from build123d import *

# Parameters (mm, degrees)
BASE_FLANGE1_DEPTH              = 0.254
EDGE_FLANGE1_STRIP_W            = 1.0668
EDGE_FLANGE1_STRIP_H            = 0.254
EDGE_FLANGE1_STRIP_CUT_DEPTH    = 6.985
EDGE_FLANGE1_RELIEF_W           = 1.1938
EDGE_FLANGE1_RELIEF_H           = 0.127
EDGE_FLANGE1_RELIEF_CUT_DEPTH   = 0.254
EDGE_FLANGE1_DEPTH              = 6.985
EDGE_FLANGE2_STRIP_W            = 1.0668
EDGE_FLANGE2_STRIP_H            = 0.254
EDGE_FLANGE2_STRIP_CUT_DEPTH    = 8.244248495
EDGE_FLANGE2_RELIEF_W           = 1.1938
EDGE_FLANGE2_RELIEF_H           = 0.127
EDGE_FLANGE2_RELIEF_CUT_DEPTH   = 0.254
EDGE_FLANGE2_STRIP_2_W          = 1.0668
EDGE_FLANGE2_STRIP_2_H          = 0.254
EDGE_FLANGE2_STRIP_CUT_2_DEPTH  = 8.244248495
EDGE_FLANGE2_RELIEF_2_W         = 1.1938
EDGE_FLANGE2_RELIEF_2_H         = 0.127
EDGE_FLANGE2_RELIEF_CUT_2_DEPTH = 0.254
EDGE_FLANGE2_DEPTH              = 8.244248495
EDGE_FLANGE2_BEND_DEPTH         = 8.244248495
EXTRUDE_THIN1_START             = -1.5875
EXTRUDE_THIN1_OUTLINE_W         = 2.8575
EXTRUDE_THIN1_OUTLINE_H         = 0.254
EXTRUDE_THIN1_DEPTH             = 3.175
CUT_EXTRUDE1_REACH              = 22.35
CUT_EXTRUDE2_REACH              = 22.35
SKETCH23_R                      = 0.508


# Read off the part's stored shape, not the designer's step: Extrude-Thin1
# Sheet-metal steps are written as plain solids
with BuildPart() as part:
    # Sketch1 → Base-Flange1 (new body)
    with BuildSketch(Plane.XY):
        with BuildLine():
            Line((3.123097979, 0), (10.108097979, 0))
            Line((10.108097979, 0), (13.219597979, 3.1115))
            Line((13.219597979, 3.1115), (13.219597979, 11.355748495))
            ThreePointArc((13.219597979, 11.355748495), (12.836917178, 11.985343025), (12.101830107, 11.935534727))
            ThreePointArc((12.101830107, 11.935534727), (6.615597979, 10.196861335), (1.129365852, 11.935534727))
            ThreePointArc((1.129365852, 11.935534727), (0.39427878, 11.985343025), (0.011597979, 11.355748495))
            Line((0.011597979, 11.355748495), (0.011597979, 3.1115))
            Line((0.011597979, 3.1115), (3.123097979, 0))
        make_face()
    extrude(amount=-BASE_FLANGE1_DEPTH)

    # Edge-Flange1 strip (across the edge) → Edge-Flange1 strip cut (cut)
    with BuildSketch(Plane(origin=(10.108097979, 0, -0.254), x_dir=(0, 1, 0), z_dir=(-1, 0, 0))):
        with Locations((-0.254, -0.127)):
            Rectangle(EDGE_FLANGE1_STRIP_W, EDGE_FLANGE1_STRIP_H)
    extrude(amount=EDGE_FLANGE1_STRIP_CUT_DEPTH, mode=Mode.SUBTRACT)

    # Edge-Flange1 relief (on the sheet) → Edge-Flange1 relief cut (cut)
    with BuildSketch(Plane(origin=(10.108097979, 0.2794, -0.254), x_dir=(0, 1, 0), z_dir=(0, 0, -1))):
        with Locations((-0.4699, 0.0635)):
            Rectangle(EDGE_FLANGE1_RELIEF_W, EDGE_FLANGE1_RELIEF_H)
        with Locations((-0.4699, -7.0485)):
            Rectangle(EDGE_FLANGE1_RELIEF_W, EDGE_FLANGE1_RELIEF_H)
    extrude(amount=-EDGE_FLANGE1_RELIEF_CUT_DEPTH, mode=Mode.SUBTRACT)

    # Edge-Flange1 section (across the edge) → Edge-Flange1 (add)
    with BuildSketch(Plane(origin=(10.108097979, 0, -0.254), x_dir=(0, 1, 0), z_dir=(-1, 0, 0))):
        with BuildLine():
            Line((0, 0.0254), (0, 1.778))
            Line((0, 1.778), (0.254, 1.778))
            Line((0.254, 1.778), (0.254, 0.0254))
            ThreePointArc((0.254, 0.0254), (0.261439488, 0.007439488), (0.2794, 0))
            Line((0.2794, 0), (0.2794, -0.254))
            ThreePointArc((0.2794, -0.254), (0.081834365, -0.172165635), (0, 0.0254))
        make_face()
    extrude(amount=EDGE_FLANGE1_DEPTH)

    # Edge-Flange2 strip (across the edge) → Edge-Flange2 strip cut (cut)
    with BuildSketch(Plane(origin=(0.011597979, 3.1115, -0.254), x_dir=(1, 0, 0), z_dir=(0, 1, 0))):
        with Locations((-0.254, -0.127)):
            Rectangle(EDGE_FLANGE2_STRIP_W, EDGE_FLANGE2_STRIP_H)
    extrude(amount=EDGE_FLANGE2_STRIP_CUT_DEPTH, mode=Mode.SUBTRACT)

    # Edge-Flange2 relief (on the sheet) → Edge-Flange2 relief cut (cut)
    with BuildSketch(Plane(origin=(0.290997979, 3.1115, -0.254), x_dir=(1, 0, 0), z_dir=(0, 0, -1))):
        with Locations((-0.4699, 0.0635)):
            Rectangle(EDGE_FLANGE2_RELIEF_W, EDGE_FLANGE2_RELIEF_H)
        with Locations((-0.4699, -8.307748495)):
            Rectangle(EDGE_FLANGE2_RELIEF_W, EDGE_FLANGE2_RELIEF_H)
    extrude(amount=-EDGE_FLANGE2_RELIEF_CUT_DEPTH, mode=Mode.SUBTRACT)

    # Edge-Flange2 strip 2 (across the edge) → Edge-Flange2 strip cut 2 (cut)
    with BuildSketch(Plane(origin=(13.219597979, 11.355748495, -0.254), x_dir=(-1, 0, 0), z_dir=(0, -1, 0))):
        with Locations((-0.254, -0.127)):
            Rectangle(EDGE_FLANGE2_STRIP_2_W, EDGE_FLANGE2_STRIP_2_H)
    extrude(amount=EDGE_FLANGE2_STRIP_CUT_2_DEPTH, mode=Mode.SUBTRACT)

    # Edge-Flange2 relief 2 (on the sheet) → Edge-Flange2 relief cut 2 (cut)
    with BuildSketch(Plane(origin=(12.940197979, 11.355748495, -0.254), x_dir=(-1, 0, 0), z_dir=(0, 0, -1))):
        with Locations((-0.4699, 0.0635)):
            Rectangle(EDGE_FLANGE2_RELIEF_2_W, EDGE_FLANGE2_RELIEF_2_H)
        with Locations((-0.4699, -8.307748495)):
            Rectangle(EDGE_FLANGE2_RELIEF_2_W, EDGE_FLANGE2_RELIEF_2_H)
    extrude(amount=-EDGE_FLANGE2_RELIEF_CUT_2_DEPTH, mode=Mode.SUBTRACT)

    # Edge-Flange2 section (across the edge) → Edge-Flange2 (add)
    with BuildSketch(Plane(origin=(0.011597979, 3.1115, -0.254), x_dir=(1, 0, 0), z_dir=(0, 1, 0))):
        with BuildLine():
            Line((0, 0.0254), (0, 2.921))
            Line((0, 2.921), (0.254, 2.921))
            Line((0.254, 2.921), (0.254, 0.0254))
            ThreePointArc((0.254, 0.0254), (0.261439488, 0.007439488), (0.2794, 0))
            Line((0.2794, 0), (0.2794, -0.254))
            ThreePointArc((0.2794, -0.254), (0.081834365, -0.172165635), (0, 0.0254))
        make_face()
    extrude(amount=EDGE_FLANGE2_DEPTH)

    # Edge-Flange2 section 2 (across the edge) → Edge-Flange2 bend (add)
    with BuildSketch(Plane(origin=(13.219597979, 11.355748495, -0.254), x_dir=(-1, 0, 0), z_dir=(0, -1, 0))):
        with BuildLine():
            Line((0, 0.0254), (0, 2.921))
            Line((0, 2.921), (0.254, 2.921))
            Line((0.254, 2.921), (0.254, 0.0254))
            ThreePointArc((0.254, 0.0254), (0.261439488, 0.007439488), (0.2794, 0))
            Line((0.2794, 0), (0.2794, -0.254))
            ThreePointArc((0.2794, -0.254), (0.081834365, -0.172165635), (0, 0.0254))
        make_face()
    extrude(amount=EDGE_FLANGE2_BEND_DEPTH)

    # Extrude-Thin1 outline → Extrude-Thin1 (add)
    with BuildSketch(Plane(origin=(0, 6.731, 0), x_dir=(-1, 0, 0), z_dir=(0, -1, 0)).offset(EXTRUDE_THIN1_START)):
        with Locations((1.417152021, 3.048)):
            Rectangle(EXTRUDE_THIN1_OUTLINE_W, EXTRUDE_THIN1_OUTLINE_H)
        with Locations((-14.648347979, 3.048)):
            Rectangle(EXTRUDE_THIN1_OUTLINE_W, EXTRUDE_THIN1_OUTLINE_H)
    extrude(amount=EXTRUDE_THIN1_DEPTH)

    # Sketch20 → Cut-Extrude1 (cut, up to next)
    with BuildSketch(Plane.XY, mode=Mode.PRIVATE) as cut_extrude1_sk1:
        with BuildLine():
            Line((2.678597979, 6.82596134), (2.678597979, 5.08))
            ThreePointArc((2.678597979, 5.08), (3.440597979, 4.318), (4.202597979, 5.08))
            Line((4.202597979, 5.08), (4.202597979, 6.82596134))
            ThreePointArc((4.202597979, 6.82596134), (3.440597979, 3.175), (2.678597979, 6.82596134))
        make_face()
    cut_extrude1_tool1 = extrude(cut_extrude1_sk1.sketch, amount=-CUT_EXTRUDE1_REACH, mode=Mode.PRIVATE) & part.part
    # Sketch20 → Cut-Extrude1 (cut, up to next)
    with BuildSketch(Plane.XY, mode=Mode.PRIVATE) as cut_extrude1_sk2:
        with BuildLine():
            Line((9.028597979, 6.82596134), (9.028597979, 5.08))
            ThreePointArc((9.028597979, 5.08), (9.790597979, 4.318), (10.552597979, 5.08))
            Line((10.552597979, 5.08), (10.552597979, 6.82596134))
            ThreePointArc((10.552597979, 6.82596134), (9.790597979, 3.175), (9.028597979, 6.82596134))
        make_face()
    cut_extrude1_tool2 = extrude(cut_extrude1_sk2.sketch, amount=-CUT_EXTRUDE1_REACH, mode=Mode.PRIVATE) & part.part
    add(cut_extrude1_tool1.solids().sort_by_distance((2.625829, 5.952981, 0))[0], mode=Mode.SUBTRACT)
    add(cut_extrude1_tool2.solids().sort_by_distance((10.605367, 5.952981, 0))[0], mode=Mode.SUBTRACT)

    # Sketch23 → Cut-Extrude2 (cut, up to next)
    with BuildSketch(Plane(origin=(0, 0, -3.175), x_dir=(-1, 0, 0), z_dir=(0, 0, -1)), mode=Mode.PRIVATE) as cut_extrude2_sk1:
        with Locations((-14.648347979, 6.731)):
            Circle(SKETCH23_R)
    cut_extrude2_tool1 = extrude(cut_extrude2_sk1.sketch, amount=-CUT_EXTRUDE2_REACH, mode=Mode.PRIVATE) & part.part
    # Sketch23 → Cut-Extrude2 (cut, up to next)
    with BuildSketch(Plane(origin=(0, 0, -3.175), x_dir=(-1, 0, 0), z_dir=(0, 0, -1)), mode=Mode.PRIVATE) as cut_extrude2_sk2:
        with Locations((1.417152021, 6.731)):
            Circle(SKETCH23_R)
    cut_extrude2_tool2 = extrude(cut_extrude2_sk2.sketch, amount=-CUT_EXTRUDE2_REACH, mode=Mode.PRIVATE) & part.part
    add(cut_extrude2_tool1.solids().sort_by_distance((14.648348, 6.731, -3.175))[0], mode=Mode.SUBTRACT)
    add(cut_extrude2_tool2.solids().sort_by_distance((-1.417152, 6.731, -3.175))[0], mode=Mode.SUBTRACT)


solid = part.part
Model file for the job. Use its own axes, mm. A direction names the side the tool comes from. Give positions to 0.01 mm unless a question says otherwise; leave off trailing zeros. Order: outer loops, then holes, each group sorted by start corner. A loop starts at its lowest first (then second) coordinate and runs counter-clockwise, first axis right, second up. Notation, with made-up numbers: (27, 3) - (31, 3) arc R33 cw to (31, 36) - close; hole circle Ø11 at (74.25, -27). An arc over 180 degrees is marked (long way). Write item = value, one per line. Start each with the question number.
1. Cut at B-B, the plane z = -0.55. List the corners of the cut face in (x, y).
2. Probe line 1 along X through (y, z) = (5.08, -0.2); line 2 along X through (y, z) = (6, -1.5); line 3 along X through (y, z) = (5.08, -0.1). List the from-to ranges inside material, lowest first.
3. Which spindle directions (+Z, -Z, +X, -X, +Y, -Y) get a long thin tool onto all of the face, cutting with end or side? Do faces 1 (the flat face through (7, 0.254, -1)), 2 (the flat face through (-1.4, 7.5, -2.921)), 3 (the flat face through (7, 0, -1)), 4 (the flat face through (14, 7, -2.921)), 5 (the flat face through (0.266, 7, -2)). Say none if no direction does.
4. Cut at A-A, the plane z = -2.6. List the corners of the cut face in (x, y), and give its area (3 significant figures).
5. Drop flat-ended pins along their axis: P1, Ø0.9, axis at y = 8, z = -1, coming from the -X side; P2, Ø1.6, axis at x = -1.42, y = 6.73, coming from the +Z side; P3, Ø1.4, axis at y = 8.5, z = -1.5, coming from the +X side. Give the stop position or say it passes through.
6. Cut at D-D, the plane y = 3.5. List the corners of the cut face in (x, z) (3 decimals), and give its area (3 significant figures).
7. Cut at C-C, the plane y = 9. List the corners of the cut face in (x, z) (3 decimals), and give its area (3 significant figures).
Taken from the geometry:
q1.outline = (0.01, 3.11) - (0.27, 3.11) - (0.27, 11.36) - (0.01, 11.36) - close; (3.12, 0) - (10.11, 0) - (10.11, 0.25) - (3.12, 0.25) - close; (12.97, 3.11) - (13.22, 3.11) - (13.22, 11.36) - (12.97, 11.36) - close
q2.line_1 = 0.02 to 1.54, 2.68 to 4.2, 5.35 to 7.89, 9.03 to 10.55, 11.7 to 13.21
q2.line_2 = 0.01 to 0.27, 12.97 to 13.22
q2.line_3 = 0.08 to 1.54, 2.68 to 4.2, 5.35 to 7.89, 9.03 to 10.55, 11.7 to 13.15
q3.face_1 = -Z, +X, -X, +Y
q3.face_2 = +Z, -X, +Y, -Y
q3.face_3 = +Z, -Z, +X, -X, -Y
q3.face_4 = +Z, +X, +Y, -Y
q3.face_5 = -Z, +Y, -Y
q4.outline = (0.01, 3.11) - (0.27, 3.11) - (0.27, 11.36) - (0.01, 11.36) - close; (12.97, 3.11) - (13.22, 3.11) - (13.22, 11.36) - (12.97, 11.36) - close
q4.area = 4.19 mm²
q5.P1 = 0.01
q5.P2 = -2.92
q5.P3 = 13.22
q6.outline = (0.012, -3.175) - (0.266, -3.175) - (0.266, -0.279) arc R0.025 cw to (0.291, -0.254) - (2.376, -0.254) - (2.376, 0) - (0.291, 0) arc R0.279 ccw to (0.012, -0.279) - close; (4.505, -0.254) - (8.726, -0.254) - (8.726, 0) - (4.505, 0) - close; (10.855, -0.254) - (12.94, -0.254) arc R0.025 cw to (12.966, -0.279) - (12.966, -3.175) - (13.22, -3.175) - (13.22, -0.279) arc R0.279 ccw to (12.94, 0) - (10.855, 0) - close
q6.area = 3.72 mm²
q7.outline = (0.012, -3.175) - (0.266, -3.175) - (0.266, -0.279) arc R0.025 cw to (0.291, -0.254) - (12.94, -0.254) arc R0.025 cw to (12.966, -0.279) - (12.966, -3.175) - (13.22, -3.175) - (13.22, -0.279) arc R0.279 ccw to (12.94, 0) - (0.291, 0) arc R0.279 ccw to (0.012, -0.279) - close
q7.area = 4.81 mm²
